Part model, mm, in its own coordinate system. Coordinates: 2 decimals unless noted, no trailing zeros. Order: outer loops, then holes, each group sorted by start corner. A loop starts at its lowest first (then second) coordinate and runs counter-clockwise, first axis right, second up. Notation, with made-up numbers: M 50,3 L 102,3 A31 cw 102,38 Z; hole C -22,42 d11. An arc over 180 degrees is marked long. Answer in a Markdown table with one row per item. Add a question column.
from build123d import *

# Parameters (mm, degrees)
SKETCH1_R           = 2.55
BOSS_EXTRUDE1_DEPTH = 4


with BuildPart() as part:
    # Sketch1 → Boss-Extrude1 (new body)
    with BuildSketch(Plane.XY):
        with BuildLine():
            Line((14.872885109, 17.599965411), (12.706250758, 42.361500851))
            Line((12.706250758, 42.361500851), (12.474619372, 45.008716695))
            Line((12.474619372, 45.008716695), (12.474619372, 47))
            Line((12.474619372, 47), (32.474619372, 47))
            Line((32.474619372, 47), (32.474619372, 45))
            Line((32.474619372, 45), (162.509181482, 14.606317485))
            ThreePointArc((162.509181482, 14.606317485), (174.095167783, 0), (162.509181482, -14.606317485))
            Line((162.509181482, -14.606317485), (32.474619372, -45))
            Line((32.474619372, -45), (32.474619372, -47))
            Line((32.474619372, -47), (12.474619372, -47))
            Line((12.474619372, -47), (12.474619372, -45.008716695))
            Line((12.474619372, -45.008716695), (12.706250758, -42.361500851))
            Line((12.706250758, -42.361500851), (14.872885109, -17.599965411))
            ThreePointArc((14.872885109, -17.599965411), (15.740145918, -15.740145918), (17.599965411, -14.872885109))
            Line((17.599965411, -14.872885109), (42.361500851, -12.706250758))
            ThreePointArc((42.361500851, -12.706250758), (44.311843411, -11.744427787), (45.1, -9.717669606))
            Line((45.1, -9.717669606), (45.1, 9.717669606))
            ThreePointArc((45.1, 9.717669606), (44.311843411, 11.744427787), (42.361500851, 12.706250758))
            Line((42.361500851, 12.706250758), (17.599965411, 14.872885109))
            ThreePointArc((17.599965411, 14.872885109), (15.740145918, 15.740145918), (14.872885109, 17.599965411))
        make_face()
        with Locations((159.095167783, 0)):
            Circle(SKETCH1_R, mode=Mode.SUBTRACT)
        with Locations((90, 0)):
            Circle(SKETCH1_R, mode=Mode.SUBTRACT)
    extrude(amount=BOSS_EXTRUDE1_DEPTH)


solid = part.part
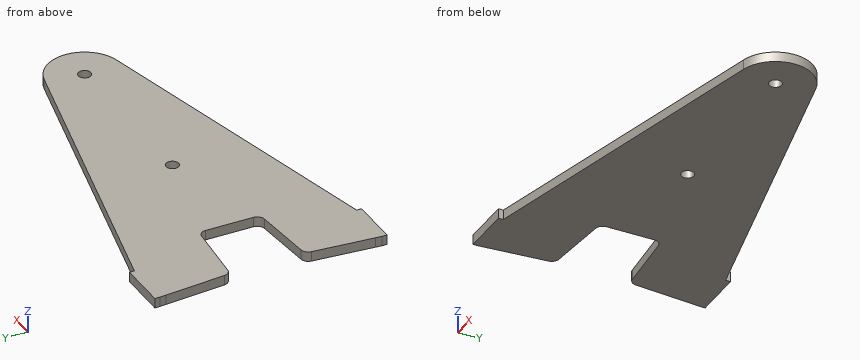
(1) Slice it at D-D (x = 36). List the corners of the cut face in (y, z), and give its area (3 significant figures).
(2) Slice it at B-B (y = 0). List the corners of the cut face in (x, z).
(3) Wall check: line 1 (Y direction, x = 90, z = 1.25); line 2 (Y direction, x = 41.5, z = 1.8); line 3 (Y direction, x = 162.5, z = 3.05). Give the ranges that are in metal, low to high.
(4) Drop a flat-ended pin along its axis: P1, Ø2, axis at y = -46.5, z = 2, coming from the +X side. Give the stop position or say it passes through.
(5) Slice it at A-A (z = 3.25). List the corners of the cut face in (x, y).
(6) Slice it at C-C (x = 90). List the corners of the cut face in (y, z), and give its area (3 significant figures).
Computed:
| question | item | result |
|---|---|---|
| 1 | outline | M -44.18,0 L -13.26,0 L -13.26,4 L -44.18,4 Z; M 13.26,0 L 44.18,0 L 44.18,4 L 13.26,4 Z |
| 1 | area | 247 mm^2 |
| 2 | outline | M 45.1,0 L 87.45,0 L 87.45,4 L 45.1,4 Z; M 92.55,0 L 156.55,0 L 156.55,4 L 92.55,4 Z; M 161.65,0 L 174.1,0 L 174.1,4 L 161.65,4 Z |
| 3 | line 1 | y = -31.55 to -2.55, 2.55 to 31.55 |
| 3 | line 2 | y = -42.89 to -12.78, 12.78 to 42.89 |
| 3 | line 3 | y = -14.61 to 14.61 |
| 4 | P1 | stops at x = 32.47 |
| 5 | outline | M 12.47,-47 L 32.47,-47 L 32.47,-45 L 162.51,-14.61 A15 ccw 162.51,14.61 L 32.47,45 L 32.47,47 L 12.47,47 L 12.47,45.01 L 14.87,17.6 A3 ccw 17.6,14.87 L 42.36,12.71 A3 cw 45.1,9.72 L 45.1,-9.72 A3 cw 42.36,-12.71 L 17.6,-14.87 A3 ccw 14.87,-17.6 L 12.47,-45.01 Z; hole C 90,0 d5.1; hole C 159.1,0 d5.1 |
| 6 | outline | M -31.55,0 L -2.55,0 L -2.55,4 L -31.55,4 Z; M 2.55,0 L 31.55,0 L 31.55,4 L 2.55,4 Z |
| 6 | area | 232 mm^2 |
